```python
from build123d import *

# Parameters (mm, degrees)
SKETCH_1_W          = 98.2
SKETCH_1_H          = 60
SKETCH_1_R          = 1.85
EXTRUDE_1_DEPTH     = 1.7
SKETCH_2_W          = 97
SKETCH_2_H          = 40
EXTRUDE_2_DEPTH     = 9.9
CUT_EXTRUDE_1_DEPTH = 0.8
EXTRUDE_START       = -2.7
SKETCH_4_W          = 42
SKETCH_4_H          = 19.6
EXTRUDE_3_DEPTH     = 1.5
SKETCH_5_W          = 40.7
SKETCH_5_H          = 2.6
EXTRUDE_4_DEPTH     = 2.7
SKETCH_6_W          = 7
SKETCH_6_H          = 7
EXTRUDE_5_DEPTH     = 5
SKETCH_6_3_W        = 7.5
SKETCH_6_3_H        = 10.5
EXTRUDE_6_DEPTH     = 2.2


with BuildPart() as part:
    # Sketch 1 → Extrude 1 (new body)
    with BuildSketch(Plane(origin=(0, 0, 0), x_dir=(1, 0, 0), z_dir=(0, 1, 0))):
        Rectangle(SKETCH_1_W, SKETCH_1_H)
        with Locations(Location((46.4, 27.4, 0), (0, 0, 270))):
            Circle(SKETCH_1_R, mode=Mode.SUBTRACT)
        with Locations(Location((-46.4, 27.4, 0), (0, 0, 90))):
            Circle(SKETCH_1_R, mode=Mode.SUBTRACT)
        with Locations(Location((46.4, -27.4, 0), (0, 0, 90))):
            Circle(SKETCH_1_R, mode=Mode.SUBTRACT)
        with Locations(Location((-46.4, -27.4, 0), (0, 0, 270))):
            Circle(SKETCH_1_R, mode=Mode.SUBTRACT)
    extrude(amount=EXTRUDE_1_DEPTH)

    # Sketch 2 → Extrude 2 (add)
    with BuildSketch(Plane(origin=(0, 0, 0), x_dir=(1, 0, 0), z_dir=(0, 1, 0))):
        with Locations((0.2, -0.1)):
            Rectangle(SKETCH_2_W, SKETCH_2_H)
    extrude(amount=EXTRUDE_2_DEPTH)

    # Sketch 3 → Cut-Extrude 1 (cut)
    with BuildSketch(Plane(origin=(0, 9.9, 0), x_dir=(1, 0, 0), z_dir=(0, 1, 0))):
        with BuildLine():
            Line((-36.9, -13.2), (37.3, -13.2))
            ThreePointArc((37.3, -13.2), (38.007106781, -12.907106781), (38.3, -12.2))
            Line((38.3, -12.2), (38.3, 12))
            ThreePointArc((38.3, 12), (38.007106781, 12.707106781), (37.3, 13))
            Line((37.3, 13), (-36.9, 13))
            ThreePointArc((-36.9, 13), (-37.607106781, 12.707106781), (-37.9, 12))
            Line((-37.9, 12), (-37.9, -12.2))
            ThreePointArc((-37.9, -12.2), (-37.607106781, -12.907106781), (-36.9, -13.2))
        make_face()
    extrude(amount=-CUT_EXTRUDE_1_DEPTH, mode=Mode.SUBTRACT)



with BuildPart() as body_2:
    # Sketch 4 → Extrude 3 (new body)
    with BuildSketch(Plane(origin=(0, 0, 0), x_dir=(1, 0, 0), z_dir=(0, 1, 0)).offset(EXTRUDE_START)):
        with Locations((-20.3, 19.1)):
            Rectangle(SKETCH_4_W, SKETCH_4_H)
    extrude(amount=-EXTRUDE_3_DEPTH)


with BuildPart() as part_1:
    add(part.part)

    add(body_2.part)  # Extrude 4 merges body 2
    # Sketch 5 → Extrude 4 (add)
    with BuildSketch(Plane(origin=(0, 0, 0), x_dir=(1, 0, 0), z_dir=(0, 1, 0))):
        with Locations((-19.95, 27.6)):
            Rectangle(SKETCH_5_W, SKETCH_5_H)
    extrude(amount=-EXTRUDE_4_DEPTH)

    # Sketch 6 → Extrude 5 (add)
    with BuildSketch(Plane.XZ.offset(4.2)):
        with Locations((-30, -21.2)):
            Rectangle(SKETCH_6_W, SKETCH_6_H)
    extrude(amount=EXTRUDE_5_DEPTH)

    # Sketch 6_3 → Extrude 6 (add)
    with BuildSketch(Plane.XZ.offset(4.2)):
        with Locations((-19.15, -20.45)):
            Rectangle(SKETCH_6_3_W, SKETCH_6_3_H)
    extrude(amount=EXTRUDE_6_DEPTH)


solid = part_1.part
```
CAD build for the part. Positions are in the model's coordinates, mm. A direction names the side the tool comes from. Coordinates: 2 decimals unless noted, no trailing zeros. Write each loop counter-clockwise with the first axis right and the second up, starting at its lowest first coordinate (ties: lowest second). Pieces come first, ordered by that corner, then holes.
(1) Two-plate mould, pull along X, no slides. Class faces 1 (the face through (-1, 0, 0)), 2 (the face through (45.844, 0.838, 25.635)), 3 (the face through (-33.5, -7, -21)), 4 (the face through (0.4, -1, -28)): +X half, -X half, draft (parallel to the pull), parting line (faces both ways), or undercut.
(2) Drill centre lines: probe 1 along X at (y, z) = (0.4, 27.4); probe 2 along Y at (x, z) = (-8.5, -20.5); probe 3 along Z at (x, y) = (13, 8). Where is each one in solid material? Low to high.
(3) Flat gauge pins, fed straight in: pin 1 (2.5 mm diameter, centred on x = -28.5, y = -5.5, fed in from +Z); pin 2 (6 mm diameter, centred on x = 6.5, z = -1.5, fed in from -Y); pin 3 (2.5 mm diameter, centred on y = -5, z = -20.5, fed in from -X). Where does each tip first touch, or does it go through?
(4) 3-axis set-ups, long thin cutter, end or side, ignore diameter. For faces 5 (the face through (-30, -7, -17.7)), 6 (the face through (-19, -5, -25.7)), 7 (the face through (-20, -1, -26.3)), 8 (the face through (48.7, 6, 0)): which of +Z, -Z, +X, -X, +Y, -Y reach the whole face in a straight line?
(5) Cut at A-A, the plane z = 27.4. List the corners of the cut face in (x, y).
(6) Cut at B-B, the plane x = -46.4. List the corners of the cut face in (y, z), and give its area (3 significant figures).
(7) Cut at C-C, the plane z = 7.5. List the corners of the cut face in (x, y), and give its area (3 significant figures).
(8) Cut at D-D, the plane x = 28. List the corners of the cut face in (y, z), and give its area (3 significant figures).
Geometry says:
1. face 1: draft
1. face 2: undercut
1. face 3: -X half
1. face 4: +X half
2. probe 1: x = -49.1 to -48.25, -44.55 to 44.55, 48.25 to 49.1
2. probe 2: y = -4.2 to -2.7, 0 to 1.7
2. probe 3: z = -19.9 to 20.1
3. pin 1: stops at z = -17.7
3. pin 2: stops at y = 0
3. pin 3: stops at x = -41.3
4. face 5: +Z, -X, -Y
4. face 6: -Z, +X, -X, -Y
4. face 7: +Z, +X, -X
4. face 8: +Z, -Z, +X, +Y
5. outline: (-49.1, 0) - (-48.25, 0) - (-48.25, 1.7) - (-49.1, 1.7) - close; (-44.55, 0) - (44.55, 0) - (44.55, 1.7) - (-44.55, 1.7) - close; (48.25, 0) - (49.1, 0) - (49.1, 1.7) - (48.25, 1.7) - close
6. outline: (0, -30) - (1.7, -30) - (1.7, -29.25) - (0, -29.25) - close; (0, -25.55) - (1.7, -25.55) - (1.7, -19.9) - (9.9, -19.9) - (9.9, 20.1) - (1.7, 20.1) - (1.7, 25.55) - (0, 25.55) - close; (0, 29.25) - (1.7, 29.25) - (1.7, 30) - (0, 30) - close
6. area: 417 mm2
7. outline: (-49.1, 0) - (49.1, 0) - (49.1, 1.7) - (48.7, 1.7) - (48.7, 9.9) - (38.3, 9.9) - (38.3, 9.1) - (-37.9, 9.1) - (-37.9, 9.9) - (-48.3, 9.9) - (-48.3, 1.7) - (-49.1, 1.7) - close
7. area: 901 mm2
8. outline: (0, -30) - (1.7, -30) - (1.7, -19.9) - (9.9, -19.9) - (9.9, -13) - (9.1, -13) - (9.1, 13.2) - (9.9, 13.2) - (9.9, 20.1) - (1.7, 20.1) - (1.7, 30) - (0, 30) - close
8. area: 409 mm2
